```python
from build123d import *

# Parameters (mm, degrees)
SKETCH1_W           = 30
SKETCH1_H           = 2.5
BOSS_EXTRUDE1_DEPTH = 1.25
FILLET1_R           = 3


with BuildPart() as part:
    # Sketch1 → Boss-Extrude1 (new, symmetric)
    with BuildSketch(Plane.XY):
        Polygon((-105, -37.5), (-105, -30), (-105, -15), (-107.5, -15), (-107.5, 15), (-105, 15), (-105, 30), (-75, 30), (-75, 32.5), (-45, 32.5), (-45, 30), (-15, 30), (-15, 32.5), (15, 32.5), (15, 30), (45, 30), (45, 32.5), (75, 32.5), (75, 30), (105, 30), (105, 15), (107.5, 15), (107.5, -15), (105, -15), (105, -30), (105, -37.5), align=None)
        with Locations((-60, -31.25)):
            Rectangle(SKETCH1_W, SKETCH1_H, mode=Mode.SUBTRACT)
        with Locations((0, -31.25)):
            Rectangle(SKETCH1_W, SKETCH1_H, mode=Mode.SUBTRACT)
        with Locations((60, -31.25)):
            Rectangle(SKETCH1_W, SKETCH1_H, mode=Mode.SUBTRACT)
    extrude(amount=BOSS_EXTRUDE1_DEPTH, both=True)

    # Fillet1
    fillet1_edges = [part.edges().sort_by_distance(p)[0] for p in [
        (105, -37.5, 0),
        (-105, -37.5, 0),
    ]]
    fillet(fillet1_edges, radius=FILLET1_R)


solid = part.part
```
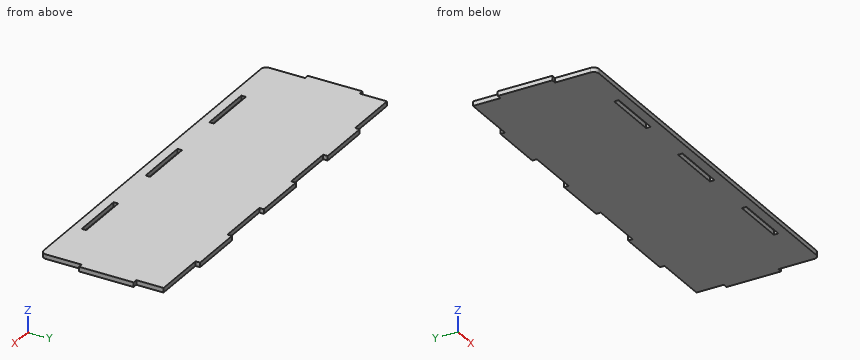
Input: part model. Units: mm. Frame: model coordinates. Give positions to 0.01 mm unless a question says otherwise; leave off trailing zeros. Order: outer loops, then holes, each group sorted by start corner. A loop starts at its lowest first (then second) coordinate and runs counter-clockwise, first axis right, second up. Notation, with made-up numbers: M 60.5,-39.5 L 98.5,-39.5 A21 ccw 98.5,-34.5 Z; hole C -38,13 d1. An arc over 180 degrees is marked long. Return JSON: item names as keys, results as strings.
1) Section query A-A on x = 54. Output: boundary loops of the cut face in (y, z).
Taken from the geometry:
{"outline": "M -37.5,-1.25 L -32.5,-1.25 L -32.5,1.25 L -37.5,1.25 Z; M -30,-1.25 L 32.5,-1.25 L 32.5,1.25 L -30,1.25 Z"}
2) Contact query for flat-ended pins moving along their axis: pin 1 (1.2 mm diameter, centred on y = -25, z = 0.5, fed in from -X); pin 2 (0.8 mm diameter, centred on x = 106, z = 0, fed in from +Y); pin 3 (0.8 mm diameter, centred on x = 91, z = -0.5, fed in from +Y). Output: stop coordinate, or through.
Taken from the geometry:
{"pin 1": "stops at x = -105", "pin 2": "stops at y = 15", "pin 3": "stops at y = 30"}
3) Section query C-C on y = 27. Output: boundary loops of the cut face in (x, z).
Taken from the geometry:
{"outline": "M -105,-1.25 L 105,-1.25 L 105,1.25 L -105,1.25 Z"}
4) Section query D-D on x = 23.5. Output: boundary loops of the cut face in (y, z).
Taken from the geometry:
{"outline": "M -37.5,-1.25 L 30,-1.25 L 30,1.25 L -37.5,1.25 Z"}
5) Line query: L1, parallel to Y at x = 6, z = -0.2; L2, parallel to Y at x = 16.5, z = -0.5; L3, parallel to X at y = 20, z = -0.75. Output: solid intervals per line, ascending. Write a range as [from, to].
Taken from the geometry:
{"L1": "y = [-37.5, -32.5], [-30, 32.5]", "L2": "y = [-37.5, 30]", "L3": "x = [-105, 105]"}
6) Section query B-B on z = -0.1. Count the separate pieces of the cut face and the enclosed holes in it, and give its area (3 significant figures).
Taken from the geometry:
{"separate pieces": "1", "enclosed holes": "3", "area": "14,300 mm2"}
